from build123d import *

# Parameters (mm, degrees)
SKETCH1_R           = 17.75
SKETCH1_W           = 23
SKETCH1_H           = 23
SKETCH1_R_2         = 1.6
BOSS_EXTRUDE1_DEPTH = 10
CUT_EXTRUDE1_START  = 10
SKETCH1_3_W         = 23
SKETCH1_3_H         = 23
SKETCH1_3_R         = 1.6
CUT_EXTRUDE1_DEPTH  = 3
SKETCH1_4_R         = 1.6
CUT_EXTRUDE3_DEPTH  = 28.020825302


with BuildPart() as part:
    # Sketch1 → Boss-Extrude1 (new body)
    # profile 1 of 6: a face of its own
    with BuildSketch(Plane(origin=(0, 0, 0), x_dir=(0, 1, 0), z_dir=(0, 0, 1))):
        with Locations(Location((0, 0, 0), (0, 0, 270))):
            Circle(SKETCH1_R)
        Rectangle(SKETCH1_W, SKETCH1_H, mode=Mode.SUBTRACT)
    # profile 2 of 6: a face of its own
    with BuildSketch(Plane(origin=(0, 0, 0), x_dir=(0, 1, 0), z_dir=(0, 0, 1))):
        Rectangle(SKETCH1_W, SKETCH1_H)
        with Locations((-8.5, -8.5)):
            Circle(SKETCH1_R_2, mode=Mode.SUBTRACT)
        with Locations((8.5, -8.5)):
            Circle(SKETCH1_R_2, mode=Mode.SUBTRACT)
        with Locations((8.5, 8.5)):
            Circle(SKETCH1_R_2, mode=Mode.SUBTRACT)
        with Locations((-8.5, 8.5)):
            Circle(SKETCH1_R_2, mode=Mode.SUBTRACT)
    # profile 3 of 6: a face of its own
    with BuildSketch(Plane(origin=(0, 0, 0), x_dir=(0, 1, 0), z_dir=(0, 0, 1))):
        with Locations((8.5, 8.5)):
            Circle(SKETCH1_R_2)
    # profile 4 of 6: a face of its own
    with BuildSketch(Plane(origin=(0, 0, 0), x_dir=(0, 1, 0), z_dir=(0, 0, 1))):
        with Locations((-8.5, 8.5)):
            Circle(SKETCH1_R_2)
    # profile 5 of 6: a face of its own
    with BuildSketch(Plane(origin=(0, 0, 0), x_dir=(0, 1, 0), z_dir=(0, 0, 1))):
        with Locations((8.5, -8.5)):
            Circle(SKETCH1_R_2)
    # profile 6 of 6: a face of its own
    with BuildSketch(Plane(origin=(0, 0, 0), x_dir=(0, 1, 0), z_dir=(0, 0, 1))):
        with Locations((-8.5, -8.5)):
            Circle(SKETCH1_R_2)
    extrude(amount=BOSS_EXTRUDE1_DEPTH)

    # Sketch1<3> → Cut-Extrude1 (cut)
    # profile 1 of 5: a face of its own
    with BuildSketch(Plane(origin=(0, 0, 0), x_dir=(0, 1, 0), z_dir=(0, 0, 1)).offset(CUT_EXTRUDE1_START)):
        Rectangle(SKETCH1_3_W, SKETCH1_3_H)
        with Locations((-8.5, -8.5)):
            Circle(SKETCH1_3_R, mode=Mode.SUBTRACT)
        with Locations((8.5, -8.5)):
            Circle(SKETCH1_3_R, mode=Mode.SUBTRACT)
        with Locations((8.5, 8.5)):
            Circle(SKETCH1_3_R, mode=Mode.SUBTRACT)
        with Locations((-8.5, 8.5)):
            Circle(SKETCH1_3_R, mode=Mode.SUBTRACT)
    # profile 2 of 5: a face of its own
    with BuildSketch(Plane(origin=(0, 0, 0), x_dir=(0, 1, 0), z_dir=(0, 0, 1)).offset(CUT_EXTRUDE1_START)):
        with Locations((-8.5, 8.5)):
            Circle(SKETCH1_3_R)
    # profile 3 of 5: a face of its own
    with BuildSketch(Plane(origin=(0, 0, 0), x_dir=(0, 1, 0), z_dir=(0, 0, 1)).offset(CUT_EXTRUDE1_START)):
        with Locations((8.5, 8.5)):
            Circle(SKETCH1_3_R)
    # profile 4 of 5: a face of its own
    with BuildSketch(Plane(origin=(0, 0, 0), x_dir=(0, 1, 0), z_dir=(0, 0, 1)).offset(CUT_EXTRUDE1_START)):
        with Locations((-8.5, -8.5)):
            Circle(SKETCH1_3_R)
    # profile 5 of 5: a face of its own
    with BuildSketch(Plane(origin=(0, 0, 0), x_dir=(0, 1, 0), z_dir=(0, 0, 1)).offset(CUT_EXTRUDE1_START)):
        with Locations((8.5, -8.5)):
            Circle(SKETCH1_3_R)
    extrude(amount=-CUT_EXTRUDE1_DEPTH, mode=Mode.SUBTRACT)

    # Sketch1<4> → Cut-Extrude3 (cut, through all)
    with BuildSketch(Plane(origin=(0, 0, 0), x_dir=(0, 1, 0), z_dir=(0, 0, 1))):
        with Locations(Location((-8.5, -8.5, 0), (0, 0, 90))):
            Circle(SKETCH1_4_R)
        with Locations(Location((8.5, -8.5, 0), (0, 0, 90))):
            Circle(SKETCH1_4_R)
        with Locations(Location((8.5, 8.5, 0), (0, 0, 90))):
            Circle(SKETCH1_4_R)
        with Locations(Location((-8.5, 8.5, 0), (0, 0, 90))):
            Circle(SKETCH1_4_R)
    extrude(amount=CUT_EXTRUDE3_DEPTH, mode=Mode.SUBTRACT)


solid = part.part
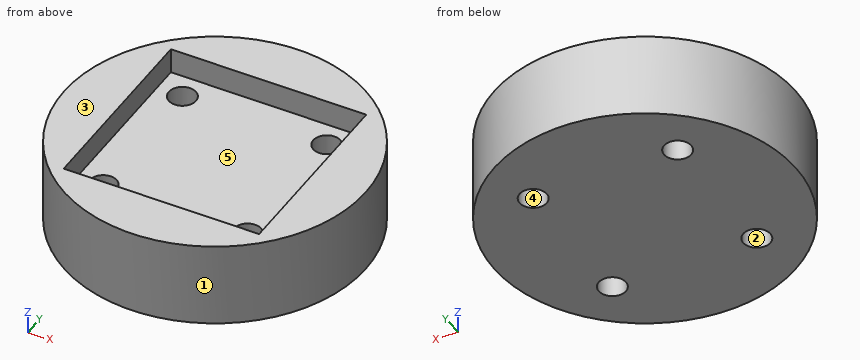
Part model, mm, in its own coordinate system. Face numbers are marked on the shaded views. A direction names the side the tool comes from. Give positions to 0.01 mm unless a question says otherwise; leave off trailing zeros. Loops run counter-clockwise (first coordinate to the right, second up) from the corner with the lowest first, then second, coordinate; pieces in that order, holes last.
(1) Drill centre lines: line 1 along X through (y, z) = (8.5, 1.5); line 2 along X through (y, z) = (9.5, 1); line 3 along Z through (x, y) = (7.5, 5). Where is each one in solid material? Low to high.
Return value:
line 1: x = -15.58 to -10.1, -6.9 to 6.9, 10.1 to 15.58
line 2: x = -14.99 to -9.75, -7.25 to 7.25, 9.75 to 14.99
line 3: z = 0 to 7
(2) Band-saw the part on A-A (y = 8.5). Write the cut outline in (x, z).
Return value:
outline: (-15.58, 0) - (-10.1, 0) - (-10.1, 7) - (-11.5, 7) - (-11.5, 10) - (-15.58, 10) - close; (-6.9, 0) - (6.9, 0) - (6.9, 7) - (-6.9, 7) - close; (10.1, 0) - (15.58, 0) - (15.58, 10) - (11.5, 10) - (11.5, 7) - (10.1, 7) - close
(3) Pull direction Y, two halves, no side cores. Call the marked faces 1, 2 and 3: pulls with the +Y half, pulls with the -Y half, needs draft (parallel to the pull), parting line crosses it, or undercut.
Return value:
face 1: parting line crosses it
face 2: undercut
face 3: needs draft
(4) 3-axis set-ups, long thin cutter, end or side, ignore diameter. For the marked faces 4 and 5: which of +Z, -Z, +X, -X, +Y, -Y reach the whole face in a straight line?
Return value:
face 4: +Z, -Z
face 5: +Z
(5) Band-saw the part on C-C (z = 5.75). Write the cut outline in (x, y), and give its area (3 significant figures).
Return value:
outline: circle Ø35.5 at (0, 0); hole circle Ø3.2 at (-8.5, -8.5); hole circle Ø3.2 at (-8.5, 8.5); hole circle Ø3.2 at (8.5, -8.5); hole circle Ø3.2 at (8.5, 8.5)
area: 958 mm2
(6) Band-saw the part on D-D (x = 0). Write the cut outline in (y, z), and give its area (3 significant figures).
Return value:
outline: (-17.75, 0) - (17.75, 0) - (17.75, 10) - (11.5, 10) - (11.5, 7) - (-11.5, 7) - (-11.5, 10) - (-17.75, 10) - close
area: 286 mm2
(7) Pin check, flat tips, straight feed: pin 1 (4 mm diameter, centred on x = -5.5, z = 6, fed in from +Y); pin 2 (5 mm diameter, centred on x = 13.5, z = 9, fed in from -Y); pin 3 (2.5 mm diameter, centred on y = 5, z = 9, fed in from -X). Stop position of each tip, or through.
Return value:
pin 1: stops at y = 17.4
pin 2: stops at y = -13.93
pin 3: stops at x = -17.35
